For this review, take the finished solid that the model builds, in its own axes (mm). Face numbers are marked on the shaded views. A direction names the side the tool comes from. Coordinates: 2 decimals unless noted, no trailing zeros. Write each loop counter-clockwise with the first axis right and the second up, starting at its lowest first coordinate (ties: lowest second). Pieces come first, ordered by that corner, then holes. Notation, with made-up numbers: (1, 63.25) -> (52, 63.25) arc R35 ccw to (52, 96.25) -> close; hole circle Ø1 at (-6, 87). An arc over 180 degrees is marked (long way). One line per item, written item: value. Start each with the question number.
1) Add section C-C (x = -4). State the section outline as (y, z) points, and give its area (3 significant figures).
2) Add section A-A (y = 0.3). State how many separate pieces and enclosed holes the cut face has, and give its area (3 significant figures).
3) For probe 1 along X at (y, z) = (0.25, -1.1); probe 2 along X at (y, z) = (0.95, -1); probe 3 along X at (y, z) = (0.45, 0.3), list the stretches that pass through material, from the lowest coordinate up. Write a range as from..to.
4) Machinability: for the marked faces 5, 6, 7, 8 and 9, which of the approach directions +Z, -Z, +X, -X, +Y, -Y give a long, thin tool a straight path to every point of the face, cutting with its end or side? Answer none if there is none.
5) Add section B-B (z = -1.15). State the section outline as (x, y) points, and give its area (3 significant figures).
6) Mouldability with a two-part tool opening along Z and no side actions: class the marked faces 1, 2, 3 and 4 as released by +Z, released by -Z, zero draft, split by the parting line, or undercut.
7) Add section D-D (z = 0.15). State the section outline as (x, y) points, and give its area (3 significant figures).
8) For pin 1 Ø1.2 at (x, z) = (4.5, -1) entering from +Y, flat-tipped, find the tip position at first contact; note if it passes through.
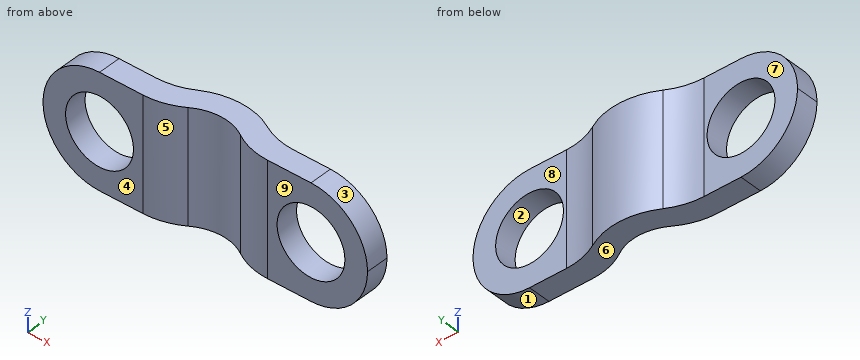
from build123d import *

# Parameters (mm, degrees)
F1_DEPTH      = 2.5
F1_DEPTH_BACK = 2.5
F2_R          = 2.49999
F3_R          = 1.5
F4_DEPTH      = 25
F5_R          = 3


# Not quite as in the source:
# - a fillet or chamfer is up to 0.001 mm smaller than in the source, because OpenCascade refuses the exact size


with BuildPart() as f1:
    # F0 (on Top) → F1 (new body, two sides)
    with BuildSketch(Plane.XY) as f1_sk:
        with BuildLine():
            Line((-6.175, 0), (-4.675, 0))
            Line((-4.675, 0), (-3.175, 0))
            Line((-3.175, 0), (-1.675, 0))
            ThreePointArc((-1.675, 0), (-0.9276877762, 0.5883021777), (0, 0.7979933839))
            Line((0, 0.7979933839), (0, 1))
            Line((0, 1), (-2.0980018512, 1))
            Line((-2.0980018512, 1), (-7.175, 1))
            Line((-7.175, 1), (-7.175, 0))
            Line((-7.175, 0), (-6.175, 0))
        make_face()
        with BuildLine():
            Line((-2.0980018512, 1), (0, 1))
            Line((0, 1), (2.0980018512, 1))
            ThreePointArc((2.0980018512, 1), (0, 1.7979933839), (-2.0980018512, 1))
        make_face()
        with BuildLine():
            Line((0, 1), (0, 0.7979933839))
            ThreePointArc((0, 0.7979933839), (0.9276877762, 0.5883021777), (1.675, 0))
            Line((1.675, 0), (3.175, 0))
            Line((3.175, 0), (4.675, 0))
            Line((4.675, 0), (6.175, 0))
            Line((6.175, 0), (7.175, 0))
            Line((7.175, 0), (7.175, 1))
            Line((7.175, 1), (2.0980018512, 1))
            Line((2.0980018512, 1), (0, 1))
        make_face()
    extrude(amount=F1_DEPTH)
    extrude(f1_sk.sketch, amount=-F1_DEPTH_BACK)

    # F2 (radius 2.5 in the source; OpenCascade refuses exactly that, so slightly less here)
    f2_edges = [f1.edges().sort_by_distance(p)[0] for p in [
        (7.175, 0.5, 2.5),
        (7.175, 0.5, -2.5),
        (-7.175, 0.5, 2.5),
        (-7.175, 0.5, -2.5),
    ]]
    fillet(f2_edges, radius=F2_R)

    # F3 (on face) → F4 (cut)
    with BuildSketch(Plane.XZ):
        with BuildLine():
            ThreePointArc((3.175, 0), (4.675, -1.5), (6.175, 0))
            ThreePointArc((6.175, 0), (4.675, 1.5), (3.175, 0))
        make_face()
        with Locations((-4.675, 0)):
            Circle(F3_R)
    extrude(amount=-F4_DEPTH, mode=Mode.SUBTRACT)

    # F5
    f5_edges = [f1.edges().sort_by_distance(p)[0] for p in [
        (1.675, 0, 0),
        (-1.675, 0, 0),
        (-2.098002, 1, 0),
        (2.098002, 1, 0),
    ]]
    fillet(f5_edges, radius=F5_R)


solid = f1.part
Numbers:
1. outline: (0, -2.5) -> (1, -2.5) -> (1, -1.34) -> (0, -1.34) -> close; (0, 1.34) -> (1, 1.34) -> (1, 2.5) -> (0, 2.5) -> close
1. area: 2.32 mm²
2. separate pieces: 2
2. enclosed holes: 2
2. area: 37.8 mm²
3. probe 1: -6.92..-5.69, -3.66..-1.56, 1.56..3.66, 5.69..6.92
3. probe 2: -6.97..-5.79, -3.56..3.56, 5.79..6.97
3. probe 3: -7.16..-6.14, -3.21..-1.18, 1.18..3.21, 6.14..7.16
4. face 5: +Z, -Z, -Y
4. face 6: -Z, +X, -X, +Y, -Y
4. face 7: +Z, -Z, -X, +Y
4. face 8: +Z, -Z, +X, +Y
4. face 9: +Z, -Z, +X, -X, -Y
5. outline: (-6.89, 0) -> (-5.64, 0) -> (-5.64, 1) -> (-6.89, 1) -> close; (-3.71, 0) -> (-2.76, 0) arc R3 ccw to (-1.15, 0.46) arc R2.16 cw to (1.15, 0.46) arc R3 ccw to (2.76, 0) -> (3.71, 0) -> (3.71, 1) -> (3.03, 1) arc R3 cw to (1.55, 1.39) arc R3.16 ccw to (-1.55, 1.39) arc R3 cw to (-3.03, 1) -> (-3.71, 1) -> close; (5.64, 0) -> (6.89, 0) -> (6.89, 1) -> (5.64, 1) -> close
5. area: 10.3 mm²
6. face 1: released by -Z
6. face 2: undercut
6. face 3: released by +Z
6. face 4: zero draft
7. outline: (-7.17, 0) -> (-6.17, 0) -> (-6.17, 1) -> (-7.17, 1) -> close; (-3.18, 0) -> (-2.76, 0) arc R3 ccw to (-1.15, 0.46) arc R2.16 cw to (1.15, 0.46) arc R3 ccw to (2.76, 0) -> (3.18, 0) -> (3.18, 1) -> (3.03, 1) arc R3 cw to (1.55, 1.39) arc R3.16 ccw to (-1.55, 1.39) arc R3 cw to (-3.03, 1) -> (-3.18, 1) -> close; (6.17, 0) -> (7.17, 0) -> (7.17, 1) -> (6.17, 1) -> close
7. area: 8.74 mm²
8. pin 1: y = 1
